CAD build for the part. Positions are in the model's coordinates, mm. Round coordinates to 2 decimals unless told otherwise and drop trailing zeros. Write each loop counter-clockwise with the first axis right and the second up, starting at its lowest first coordinate (ties: lowest second). Pieces come first, ordered by that corner, then holes. Notation, with made-up numbers: (1.5, -21) - (12.5, -21) arc R6 ccw to (12.5, -15) - close; hole circle Ø5 at (-16.5, -6.5). An arc over 180 degrees is marked (long way). Put each result on its own line as item: value. Start each with the question number.
Item 1: Cut at B-B (z = -10). Give the cut face in (x, y), and give its area (3 significant figures).
Item 2: Cut at C-C (x = 4.65). Give the cut face in (y, z).
Item 3: Mould opens along Y. For faces 1 (the cylindrical face through (2.46, -2.44, 0.54)), 2 (the cylindrical face through (2.46, 14.88, -9.46)), 3 (the cylindrical face through (2, -4, 3)), 4 (the flat face through (0, 9, -5)) say: released by +Y, released by -Y, zero draft, split by the parting line, or undercut.
Item 4: Cut at D-D (z = -13.25). Give the cut face in (x, y).
Item 5: Pin check, flat tips, straight feed: pin 1 Ø2 at (x, z) = (1, -1.5) entering from +Y; pin 2 Ø3 at (x, y) = (0.5, 11) entering from +Z. Stop position of each tip, or through.
Item 6: Drill centre lines: line 1 (Z direction, x = 2.25, y = 17); line 2 (Z direction, x = 3.3, y = -0.5); line 3 (Y direction, x = 1.7, z = 0). Where is each one in solid material? Low to high. Write a range as from..to.
Item 7: Cut at A-A (y = 19). Give the cut face in (x, z), and give its area (3 significant figures).
```python
from build123d import *

# Parameters (mm, degrees)
SKETCH1_R           = 5
SKETCH1_R_2         = 2.5
BOSS_EXTRUDE1_DEPTH = 5


with BuildPart() as part:
    # Sketch1 → Boss-Extrude1 (new body)
    # profile 1 of 3: a face of its own
    with BuildSketch(Plane(origin=(0, 0, 0), x_dir=(0, 0, -1), z_dir=(1, 0, 0))):
        with BuildLine():
            Line((5.669872981, 19.820508076), (-4.330127019, 2.5))
            ThreePointArc((-4.330127019, 2.5), (1.294095226, 4.829629131), (5, 0))
            ThreePointArc((5, 0), (4.829629131, -1.294095226), (4.330127019, -2.5))
            Line((4.330127019, -2.5), (14.330127019, 14.820508076))
            ThreePointArc((14.330127019, 14.820508076), (7.5, 12.990381057), (5.669872981, 19.820508076))
        make_face()
    # profile 2 of 3: a face of its own
    with BuildSketch(Plane(origin=(0, 0, 0), x_dir=(0, 0, -1), z_dir=(1, 0, 0))):
        with Locations((10, 17.320508076)):
            Circle(SKETCH1_R)
        with Locations((10, 17.320508076)):
            Circle(SKETCH1_R_2, mode=Mode.SUBTRACT)
    # profile 3 of 3: a face of its own
    with BuildSketch(Plane(origin=(0, 0, 0), x_dir=(0, 0, -1), z_dir=(1, 0, 0))):
        Circle(SKETCH1_R)
        Circle(SKETCH1_R_2, mode=Mode.SUBTRACT)
    extrude(amount=BOSS_EXTRUDE1_DEPTH)


solid = part.part
```
Output values:
1. outline: (0, 7.32) - (5, 7.32) - (5, 14.82) - (0, 14.82) - close; (0, 19.82) - (5, 19.82) - (5, 22.32) - (0, 22.32) - close
1. area: 50.0 mm2
2. outline: (-2.5, -4.33) - (14.82, -14.33) arc R5 ccw to (19.82, -5.67) - (2.5, 4.33) arc R5 ccw to start; hole circle Ø5 at (0, 0); hole circle Ø5 at (17.32, -10)
3. face 1: undercut
3. face 2: undercut
3. face 3: split by the parting line
3. face 4: zero draft
4. outline: (0, 12.95) - (5, 12.95) - (5, 21.12) - (0, 21.12) - close
5. pin 1: y = 14.33
5. pin 2: z = 0.29
6. line 1: -14.99..-12.48, -7.52..-4.04
6. line 2: -5.48..-2.45, 2.45..4.97
6. line 3: -5..-2.5, 2.5..10
7. outline: (0, -14.71) - (5, -14.71) - (5, -11.85) - (0, -11.85) - close; (0, -8.15) - (5, -8.15) - (5, -5.2) - (0, -5.2) - close
7. area: 29.0 mm2
